from build123d import *

# Parameters (mm, degrees)
F0_W     = 11.3675408065
F0_H     = 11.9504919276
F0_W_2   = 11.3675370812
F0_H_2   = 11.9504933245
F1_DEPTH = 21.336
F2_W     = 48.9678680897
F2_H     = 38.7662313879
F3_DEPTH = 12.7
F4_W     = 8.7442621589
F4_H     = 11.9504933245
F4_H_2   = 11.659016367
F4_W_2   = 8.1613156945
F4_H_3   = 11.6590172984
F4_W_3   = 9.3272179365
F4_H_4   = 11.9504923932
F5_DEPTH = 27.432
F6_R     = 10.3791447845
F7_DEPTH = 76.2


with BuildPart() as f1:
    # F0 (on Top) → F1 (new body)
    with BuildSketch(Plane.XY):
        Polygon((-34.1026224196, -7.1411477402), (-34.1026224196, -19.0916396677), (40.2236096561, -19.0916396677), (40.2236096561, -7.1411477402), (40.2236096561, 7.7240983956), (40.2236096561, 19.6745917201), (-34.1026224196, 19.6745917201), (-34.1026224196, 7.7240983956), align=None)
        with Locations((-39.7863928229, -13.116393704)):
            Rectangle(F0_W, F0_H)
        with Locations((45.9073781967, -13.116393704)):
            Rectangle(F0_W_2, F0_H)
        with Locations((-39.7863928229, 13.6993450578)):
            Rectangle(F0_W, F0_H_2)
        with Locations((45.9073781967, 13.6993450578)):
            Rectangle(F0_W_2, F0_H_2)
    extrude(amount=F1_DEPTH)

    # F2 (on face) → F3 (join)
    with BuildSketch(Plane.XY.offset(21.336)):
        with Locations((4.0806550533, 0.2914760262)):
            Rectangle(F2_W, F2_H)
    extrude(amount=F3_DEPTH)

    # F4 (on face) → F5 (join)
    with BuildSketch(Plane.XY.offset(21.336)):
        with Locations((-24.775410071, 13.6993450578)):
            Rectangle(F4_W, F4_H)
        with Locations((-24.775410071, -13.2621314842)):
            Rectangle(F4_W, F4_H_2)
        with Locations((33.5196731612, 13.5536070447)):
            Rectangle(F4_W_2, F4_H_3)
        with Locations((32.9367220402, -13.4078694973)):
            Rectangle(F4_W_3, F4_H_4)
    extrude(amount=F5_DEPTH)

    # F6 (on face) → F7 (cut)
    with BuildSketch(Plane.XY.offset(34.036)):
        with Locations((6.2667215243, 0)):
            Circle(F6_R)
    extrude(amount=-F7_DEPTH, mode=Mode.SUBTRACT)


solid = f1.part
Design review of the part built by this model. Coordinates are the model's own, in mm. A direction names the side the tool comes from. Round coordinates to 2 decimals unless told otherwise and drop trailing zeros. Write each loop counter-clockwise with the first axis right and the second up, starting at its lowest first coordinate (ties: lowest second). Pieces come first, ordered by that corner, then holes. Notation, with made-up numbers: (86.5, -26) -> (107.5, -26) arc R7 ccw to (107.5, -19) -> close; hole circle Ø10 at (-6.75, 16). An arc over 180 degrees is marked (long way). One line per item, written item: value. Start each with the question number.
Q1. Add section D-D (x = 14). Give the boundary of the cut face in (y, z).
Q2. Tool access review of faces 1 (the face through (40.224, 0, 11)), 2 (the face through (-40, -7.141, 11)), 3 (the face through (29.439, 13, 35)), 4 (the face through (-29.148, 14, 35)): name each direction out of +Z, -Z, +X, -X, +Y, -Y from which nothing blocks a thin tool from reaching the whole face with its end or side.
Q3. Add section A-A (z = 32). Give the boundary of the cut face in (x, y).
Q4. Insertion check: P1, Ø12, axis at y = -14, z = 32.5, coming from the -X side; P2, Ø4.5, axis at y = -2.5, z = 15, coming from the -X side; P3, Ø2, axis at x = 25, y = 6, coming from the -Z side; P4, Ø2.5, axis at x = -23.5, z = 41.5, coming from the -Y side. Each pin has a flat end and moves straight along its axis. Give the tip position at first contact, or say it passes through.
Q5. To check wall thickness, follow probe 1 along X at (y, z) = (16, 40.5); probe 2 along Y at (x, z) = (-36, 7.5); probe 3 along Y at (x, z) = (34.5, 21.5). State the ranges of each line that lie inside material, in increasing order.
Q6. Add section B-B (y = 0). Give the boundary of the cut face in (x, z).
Q7. Add section C-C (x = -25). Give the boundary of the cut face in (y, z), then the cut area to 3 significant figures.
Q8. The part is to be moulded in two halves that separate along X. For faces 5 (the face through (28.273, -13, 41)), 6 (the face through (33, 7.724, 35)), 7 (the face through (-45.47, 14, 11)), say which applies: pulls with the +X half, pulls with the -X half, needs draft (parallel to the pull), parting line crosses it, or undercut.
Response:
1. outline: (-19.09, 0) -> (-6.92, 0) -> (-6.92, 34.04) -> (-19.09, 34.04) -> close; (6.92, 0) -> (19.67, 0) -> (19.67, 34.04) -> (6.92, 34.04) -> close
2. face 1: +Z, -Z, +X
2. face 2: +Z, -Z, -X
2. face 3: +Z, +Y
2. face 4: +Z, -X, +Y, -Y
3. outline: (-29.15, -19.09) -> (28.27, -19.09) -> (28.27, -19.38) -> (37.6, -19.38) -> (37.6, -7.43) -> (28.56, -7.43) -> (28.56, 19.67) -> (-29.15, 19.67) -> (-29.15, 7.72) -> (-20.4, 7.72) -> (-20.4, -7.43) -> (-29.15, -7.43) -> close; (29.44, 7.72) -> (37.6, 7.72) -> (37.6, 19.38) -> (29.44, 19.38) -> close; hole circle Ø20.76 at (6.27, 0)
4. P1: stops at x = -29.15
4. P2: stops at x = -34.1
4. P3: stops at z = 0
4. P4: stops at y = -19.09
5. probe 1: x = -29.15 to -20.4, 29.44 to 37.6
5. probe 2: y = -19.09 to -7.14, 7.72 to 19.67
5. probe 3: y = -19.38 to -7.43, 7.72 to 19.38
6. outline: (-34.1, 0) -> (-4.11, 0) -> (-4.11, 34.04) -> (-20.4, 34.04) -> (-20.4, 21.34) -> (-34.1, 21.34) -> close; (16.65, 0) -> (40.22, 0) -> (40.22, 21.34) -> (28.56, 21.34) -> (28.56, 34.04) -> (16.65, 34.04) -> close
7. outline: (-19.09, 0) -> (19.67, 0) -> (19.67, 48.77) -> (7.72, 48.77) -> (7.72, 21.34) -> (-7.43, 21.34) -> (-7.43, 48.77) -> (-19.09, 48.77) -> close
7. area: 1,470 mm^2
8. face 5: undercut
8. face 6: needs draft
8. face 7: pulls with the -X half
